Read the model definition and answer for the solid it produces. Units are mm, in the model's axes. A direction names the side the tool comes from. Give positions to 0.01 mm unless a question says otherwise; leave off trailing zeros. Write each loop counter-clockwise with the first axis right and the second up, starting at its lowest first coordinate (ties: lowest second). Pieces come first, ordered by that corner, then holes. Notation, with made-up numbers: (35.5, 0) -> (93.5, 0) arc R28 cw to (93.5, 21) -> close; hole circle Ø3 at (-1.75, 38.25). An arc over 180 degrees is marked (long way). Use a Markdown table: item, result.
from build123d import *

# Parameters (mm, degrees)
F0_R     = 1.9
F0_R_2   = 3.1
F1_DEPTH = 3
F0_R_3   = 1.65
F2_DEPTH = 0.75
F0_R_4   = 0.9
F3_DEPTH = 7
F4_R     = 3


with BuildPart() as f1:
    # F0 (on Top) → F1 (new body)
    with BuildSketch(Plane.XY):
        with BuildLine():
            ThreePointArc((-16.75, 26.5), (-18.164214, 25.914214), (-18.75, 24.5))
            Line((-18.75, 24.5), (-18.75, -15.5))
            ThreePointArc((-18.75, -15.5), (-18.164214, -16.914214), (-16.75, -17.5))
            Line((-16.75, -17.5), (16.75, -17.5))
            ThreePointArc((16.75, -17.5), (18.164214, -16.914214), (18.75, -15.5))
            Line((18.75, -15.5), (18.75, 24.5))
            ThreePointArc((18.75, 24.5), (18.164214, 25.914214), (16.75, 26.5))
            Line((16.75, 26.5), (-16.75, 26.5))
        make_face()
        with Locations((-12, -14)):
            Circle(F0_R, mode=Mode.SUBTRACT)
        with Locations((-15.25, -7.5)):
            Circle(F0_R_2, mode=Mode.SUBTRACT)
        with Locations((12, -14)):
            Circle(F0_R, mode=Mode.SUBTRACT)
        with Locations((15.25, -7.5)):
            Circle(F0_R_2, mode=Mode.SUBTRACT)
        with Locations((-12, 14)):
            Circle(F0_R, mode=Mode.SUBTRACT)
        with Locations((-15.25, 23)):
            Circle(F0_R_2, mode=Mode.SUBTRACT)
        Polygon((-9, 11), (-9, 14), (-9, 23), (9, 23), (9, 14), (9, 11), (15.25, 11), (15.25, -2.5), (9.75, -2.5), (9, -2.5), (9, -14), (-9, -14), (-9, -2.5), (-9.75, -2.5), (-15.25, -2.5), (-15.25, 11), align=None, mode=Mode.SUBTRACT)
        with Locations((12, 14)):
            Circle(F0_R, mode=Mode.SUBTRACT)
        with Locations((15.25, 23)):
            Circle(F0_R_2, mode=Mode.SUBTRACT)
    extrude(amount=F1_DEPTH)

    # F0 (on Top) → F2 (join)
    with BuildSketch(Plane.XY):
        with Locations((-15.25, 23)):
            Circle(F0_R_2)
        with Locations((-15.25, 23)):
            Circle(F0_R_3, mode=Mode.SUBTRACT)
        with Locations((15.25, 23)):
            Circle(F0_R_2)
        with Locations((15.25, 23)):
            Circle(F0_R_3, mode=Mode.SUBTRACT)
        with Locations((15.25, -7.5)):
            Circle(F0_R_2)
        with Locations((15.25, -7.5)):
            Circle(F0_R_3, mode=Mode.SUBTRACT)
        with Locations((-15.25, -7.5)):
            Circle(F0_R_2)
        with Locations((-15.25, -7.5)):
            Circle(F0_R_3, mode=Mode.SUBTRACT)
    extrude(amount=F2_DEPTH)

    # F0 (on Top) → F3 (join)
    with BuildSketch(Plane.XY):
        with Locations((-12, 14)):
            Circle(F0_R)
        with Locations((-12, 14)):
            Circle(F0_R_4, mode=Mode.SUBTRACT)
        with Locations((12, 14)):
            Circle(F0_R)
        with Locations((12, 14)):
            Circle(F0_R_4, mode=Mode.SUBTRACT)
        with Locations((12, -14)):
            Circle(F0_R)
        with Locations((12, -14)):
            Circle(F0_R_4, mode=Mode.SUBTRACT)
        with Locations((-12, -14)):
            Circle(F0_R)
        with Locations((-12, -14)):
            Circle(F0_R_4, mode=Mode.SUBTRACT)
    extrude(amount=F3_DEPTH)

    # F4
    f4_edges = [f1.edges().sort_by_distance(p)[0] for p in [
        (-15.25, 11, 1.5),
        (-9, 23, 1.5),
        (-9, 11, 1.5),
        (9, 23, 1.5),
        (9, 11, 1.5),
        (15.25, 11, 1.5),
        (15.25, -2.5, 1.5),
        (9, -2.5, 1.5),
        (9, -14, 1.5),
        (-9, -2.5, 1.5),
        (-9, -14, 1.5),
        (-15.25, -2.5, 1.5),
    ]]
    fillet(f4_edges, radius=F4_R)


solid = f1.part
Item 1: For a pull along Y with two mould halves and no side action, classify faces 1 (the face through (18.18, 25.9, 1.48)), 2 (the face through (18.15, -16.93, 1.48)), 3 (the face through (-14.39, -1.6, 1.52)) as +Y half, -Y half, draft (parallel to the pull), parting line (faces both ways), or undercut.
Return value:
| item | result |
|---|---|
| face 1 | +Y half |
| face 2 | -Y half |
| face 3 | undercut |
Item 2: A cutting plane is placed at C-C (y = 2). Give the vertices of the cut face in (x, z), then the cut area to 3 significant figures.
Return value:
| item | result |
|---|---|
| outline | (-18.75, 0) -> (-15.25, 0) -> (-15.25, 3) -> (-18.75, 3) -> close; (15.25, 0) -> (18.75, 0) -> (18.75, 3) -> (15.25, 3) -> close |
| area | 21.0 mm^2 |
Item 3: A cutting plane is placed at A-A (z = 4). Give the vertices of the cut face in (x, y).
Return value:
| item | result |
|---|---|
| outline | circle Ø3.8 at (-12, -14); circle Ø3.8 at (-12, 14); circle Ø3.8 at (12, -14); circle Ø3.8 at (12, 14); hole circle Ø1.8 at (-12, -14); hole circle Ø1.8 at (-12, 14); hole circle Ø1.8 at (12, -14); hole circle Ø1.8 at (12, 14) |
Item 4: A tool of negligible diameter and unlimited length cuts with its end or side. For faces 4 (the face through (-11.123, 12.314, 4.972)), 5 (the face through (-18.15, 25.93, 1.48)), 6 (the face through (-9.9, 11.86, 1.52)), from which of +Z, -Z, +X, -X, +Y, -Y can it reach the whole face along a straight path? Write none if from no direction.
Return value:
| item | result |
|---|---|
| face 4 | +Z |
| face 5 | +Z, -Z, -X, +Y |
| face 6 | +Z, -Z |
Item 5: Straight lines are drawn through the part: line 1 along Y through (x, z) = (-12, 1.75); line 2 along Y through (x, z) = (-3.5, 2); line 3 along Y through (x, z) = (-12, 4.75). For each, find the intervals that lie inside material, in ascending order. Write a range as [from, to].
Return value:
| item | result |
|---|---|
| line 1 | [-17.5, -14.9], [-13.1, -2.5], [11, 13.1], [14.9, 26.5] |
| line 2 | [-17.5, -14], [23, 26.5] |
| line 3 | [-15.9, -14.9], [-13.1, -12.1], [12.1, 13.1], [14.9, 15.9] |
Item 6: A cutting plane is placed at B-B (y = -7.5). Give the vertices of the cut face in (x, z), then the cut area to 4 significant figures.
Return value:
| item | result |
|---|---|
| outline | (-18.75, 0) -> (-16.9, 0) -> (-16.9, 0.75) -> (-18.35, 0.75) -> (-18.35, 3) -> (-18.75, 3) -> close; (-13.6, 0) -> (-9, 0) -> (-9, 3) -> (-12.15, 3) -> (-12.15, 0.75) -> (-13.6, 0.75) -> close; (9, 0) -> (13.6, 0) -> (13.6, 0.75) -> (12.15, 0.75) -> (12.15, 3) -> (9, 3) -> close; (16.9, 0) -> (18.75, 0) -> (18.75, 3) -> (18.35, 3) -> (18.35, 0.75) -> (16.9, 0.75) -> close |
| area | 25.65 mm^2 |
Item 7: Each of these flat-tipped pins is pushed along its axis until it touches: P1, Ø5, axis at x = 14.5, y = 23.5, coming from the +Z side; P2, Ø4, axis at x = 15.25, y = -7.5, coming from the +Z side. Where does it stop, or does it pass through?
Return value:
| item | result |
|---|---|
| P1 | z = 3 |
| P2 | z = 0.75 |
